Verification items for the finished model (mm, model axes). A direction names the side the tool comes from. Coordinates: 2 decimals unless noted, no trailing zeros. Write each loop counter-clockwise with the first axis right and the second up, starting at its lowest first coordinate (ties: lowest second). Pieces come first, ordered by that corner, then holes. Notation, with made-up numbers: (53, 80) -> (98, 80) arc R13 ccw to (98, 91) -> close; hole circle Ø4 at (-29, 2.5). An arc over 180 degrees is marked (long way). Answer in a Markdown table with one row per item.
```python
from build123d import *

# Parameters (mm, degrees)
SKETCH1_R           = 1
BOSS_EXTRUDE1_DEPTH = 10
SKETCH2_W           = 3
SKETCH2_H           = 2
BOSS_EXTRUDE2_DEPTH = 10
FILLET1_R           = 3
SKETCH3_W           = 4
SKETCH3_H           = 3
BOSS_EXTRUDE3_DEPTH = 2
FILLET2_R           = 0.5


with BuildPart() as part:
    # Sketch1 → Boss-Extrude1 (new body)
    with BuildSketch(Plane.XY):
        with BuildLine():
            Line((5.55, -2), (-5.55, -2))
            ThreePointArc((-5.55, -2), (-7.55, 0), (-5.55, 2))
            Line((-5.55, 2), (5.55, 2))
            ThreePointArc((5.55, 2), (7.55, 0), (5.55, -2))
        make_face()
        with Locations((-5.55, 0)):
            Circle(SKETCH1_R, mode=Mode.SUBTRACT)
        with Locations((5.55, 0)):
            Circle(SKETCH1_R, mode=Mode.SUBTRACT)
    extrude(amount=BOSS_EXTRUDE1_DEPTH)

    # Sketch2 → Boss-Extrude2 (add)
    with BuildSketch(Plane(origin=(0, 2, 0), x_dir=(1, 0, 0), z_dir=(0, 1, 0))):
        with Locations((0, -5)):
            Rectangle(SKETCH2_W, SKETCH2_H)
    extrude(amount=BOSS_EXTRUDE2_DEPTH)

    # Fillet1
    fillet1_edges = [part.edges().sort_by_distance(p)[0] for p in [
        (1.5, 2, 5),
        (0, 2, 4),
        (-1.5, 2, 5),
        (0, 2, 6),
    ]]
    fillet(fillet1_edges, radius=FILLET1_R)

    # Sketch3 → Boss-Extrude3 (add)
    with BuildSketch(Plane(origin=(0, 12, 0), x_dir=(1, 0, 0), z_dir=(0, 1, 0))):
        with Locations((0, -5)):
            Rectangle(SKETCH3_W, SKETCH3_H)
    extrude(amount=BOSS_EXTRUDE3_DEPTH)

    # Fillet2
    fillet2_edges = [part.edges().sort_by_distance(p)[0] for p in [
        (1.5, 12, 5),
        (0, 12, 4),
        (-1.5, 12, 5),
        (0, 12, 6),
        (-2, 14, 5),
        (0, 14, 6.5),
        (2, 14, 5),
        (0, 14, 3.5),
    ]]
    fillet(fillet2_edges, radius=FILLET2_R - 0.0001)  # a hair under: the kernel refuses the full size


solid = part.part
```
1. Access from +Z, -Z, +X, -X, +Y, -Y to the whole of each face (thin tool, end or side, straight path). Record for faces 1 (the face through (-2, 13, 5)), 2 (the face through (0.06, 2.52, 2.69)), 3 (the face through (-0.1, 2, 9.4)), 4 (the face through (0, 13, 3.5)), 5 (the face through (0, 8, 6)).
Findings below:
| item | result |
|---|---|
| face 1 | +Z, -Z, -X, +Y |
| face 2 | -Z, +X, -X |
| face 3 | +Y |
| face 4 | -Z, +X, -X, +Y |
| face 5 | +Z, +X, -X |
2. Sectioned sample at A-A, the plane y = 0. Record the cut outline in (x, z).
Findings below:
| item | result |
|---|---|
| outline | (-7.55, 0) -> (-6.55, 0) -> (-6.55, 10) -> (-7.55, 10) -> close; (-4.55, 0) -> (4.55, 0) -> (4.55, 10) -> (-4.55, 10) -> close; (6.55, 0) -> (7.55, 0) -> (7.55, 10) -> (6.55, 10) -> close |
3. Sectioned sample at D-D, the plane z = 7.75. Record the cut outline in (x, y), and give its area (3 significant figures).
Findings below:
| item | result |
|---|---|
| outline | (-5.55, -2) -> (5.55, -2) arc R2 ccw to (5.55, 2) -> (4.5, 2) arc R3 cw to (3.25, 2.27) -> (-3.25, 2.27) arc R3 cw to (-4.5, 2) -> (-5.55, 2) arc R2 ccw to start; hole circle Ø2 at (-5.55, 0); hole circle Ø2 at (5.55, 0) |
| area | 52.7 mm² |
4. Go/stop test with flat-tipped pins: pin 1 (3.5 mm diameter, centred on x = 0.5, y = 7, fed in from -Z); pin 2 (3.5 mm diameter, centred on x = 0.5, y = 7, fed in from +Z); pin 3 (1 mm diameter, centred on y = 8, z = 5, fed in from -X). Record where each tip stops, or that it passes through.
Findings below:
| item | result |
|---|---|
| pin 1 | stops at z = 4 |
| pin 2 | stops at z = 6 |
| pin 3 | stops at x = -1.5 |
5. Release check for a two-part mould opening along X. For faces 6 (the face through (4.55, 0.04, 4.93)), 7 (the face through (1.5, 8, 5)), 8 (the face through (-2.81, 2.52, 4.94)) record: released by +X, released by -X, zero draft, split by the parting line, or undercut.
Findings below:
| item | result |
|---|---|
| face 6 | undercut |
| face 7 | released by +X |
| face 8 | released by -X |
6. Material ranges on probe 1 along Y at (x, z) = (-5.55, 7.25); probe 2 along X at (y, z) = (-0.5, 7); probe 3 along X at (y, z) = (11.5, 5.75), recorded low to high. Write a range as from..to.
Findings below:
| item | result |
|---|---|
| probe 1 | y = -2..-1, 1..2 |
| probe 2 | x = -7.49..-6.42, -4.68..4.68, 6.42..7.49 |
| probe 3 | x = -1.5..1.5 |
7. Sectioned sample at C-C, the plane x = 5. Record the cut outline in (y, z).
Findings below:
| item | result |
|---|---|
| outline | (-2, 0) -> (-0.84, 0) -> (-0.84, 10) -> (-2, 10) -> close; (0.84, 0) -> (2, 0) -> (2, 10) -> (0.84, 10) -> close |
